Design review of the part built by this model. Coordinates are the model's own, in mm. A direction names the side the tool comes from. Coordinates: 2 decimals unless noted, no trailing zeros. Loops run counter-clockwise (first coordinate to the right, second up) from the corner with the lowest first, then second, coordinate; pieces in that order, holes last. Notation, with made-up numbers: (3, 85) -> (46, 85) arc R13 cw to (46, 100) -> close; hole circle Ø11 at (20.5, -11.75). An arc over 180 degrees is marked (long way). Answer in a Markdown table with one row per item.
```python
from build123d import *

# Parameters (mm, degrees)
BOSS_EXTRU_1_DEPTH      = 8.5
BOSS_EXTRU_1_DEPTH_BACK = 8.5
D_GAGEMENT_M41_D        = 4.8


with BuildPart() as part:
    # Esquisse1 → Boss.-Extru.1 (new, two sides: drawn at the far end of the back side and taken through both)
    with BuildSketch(Plane(origin=(0, 0, 0), x_dir=(0, 0, -1), z_dir=(1, 0, 0)).offset(-BOSS_EXTRU_1_DEPTH_BACK)):
        with BuildLine():
            Line((-3.307189139, 3.75), (-11.307189139, 3.75))
            Line((-11.307189139, 3.75), (-11.307189139, 1.75))
            Line((-11.307189139, 1.75), (-0.968245837, 1.75))
            ThreePointArc((-0.968245837, 1.75), (2, 0), (-0.968245837, -1.75))
            Line((-0.968245837, -1.75), (-11.307189139, -1.75))
            Line((-11.307189139, -1.75), (-11.307189139, -3.75))
            Line((-11.307189139, -3.75), (-3.307189139, -3.75))
            ThreePointArc((-3.307189139, -3.75), (5, 0), (-3.307189139, 3.75))
        make_face()
    extrude(amount=BOSS_EXTRU_1_DEPTH + BOSS_EXTRU_1_DEPTH_BACK)

    # Dégagement M41 (through all)
    with Locations(Plane(origin=(0, 3.75, 0), x_dir=(1, 0, 0), z_dir=(0, 1, 0))):
        with Locations((0, -7.307189139)):
            Hole(D_GAGEMENT_M41_D / 2)


solid = part.part
```
(1) Take a section at D-D on z = 0. Give the boundary of the cut face in (x, y).
Evaluation:
| item | result |
|---|---|
| outline | (-8.5, -5) -> (8.5, -5) -> (8.5, -2) -> (-8.5, -2) -> close; (-8.5, 2) -> (8.5, 2) -> (8.5, 5) -> (-8.5, 5) -> close |
(2) Take a section at B-B on z = 10.25. Give the boundary of the cut face in (x, y).
Evaluation:
| item | result |
|---|---|
| outline | (-8.5, -3.75) -> (8.5, -3.75) -> (8.5, -1.75) -> (-8.5, -1.75) -> close; (-8.5, 1.75) -> (8.5, 1.75) -> (8.5, 3.75) -> (-8.5, 3.75) -> close |
(3) Take a section at C-C on x = 4.5. Give the boundary of the cut face in (y, z), and give its area (3 significant figures).
Evaluation:
| item | result |
|---|---|
| outline | (-3.75, 3.31) arc R5 ccw (long way) to (3.75, 3.31) -> (3.75, 11.31) -> (1.75, 11.31) -> (1.75, 0.97) arc R2 cw (long way) to (-1.75, 0.97) -> (-1.75, 11.31) -> (-3.75, 11.31) -> close |
| area | 83.6 mm² |
(4) Take a section at A-A on x = 0. Give the boundary of the cut face in (y, z).
Evaluation:
| item | result |
|---|---|
| outline | (-3.75, 3.31) arc R5 ccw (long way) to (3.75, 3.31) -> (3.75, 4.91) -> (1.75, 4.91) -> (1.75, 0.97) arc R2 cw (long way) to (-1.75, 0.97) -> (-1.75, 4.91) -> (-3.75, 4.91) -> close; (-3.75, 9.71) -> (-1.75, 9.71) -> (-1.75, 11.31) -> (-3.75, 11.31) -> close; (1.75, 9.71) -> (3.75, 9.71) -> (3.75, 11.31) -> (1.75, 11.31) -> close |
(5) For pin 1 (8.5 mm diameter, centred on x = 0.5, z = 5, fed in from +Y); pin 2 (4 mm diameter, centred on x = -4, z = 9.5, fed in from -Y), all flat-tipped, find the tip position at first contact; note any pin that passes through.
Evaluation:
| item | result |
|---|---|
| pin 1 | stops at y = 4.94 |
| pin 2 | stops at y = -3.75 |
(6) To check wall thickness, follow probe 1 along Y at (x, z) = (0, 0); probe 2 along Y at (x, z) = (1.5, 4); probe 3 along X at (y, z) = (-3, 6). State the ranges of each line that lie inside material, in increasing order.
Evaluation:
| item | result |
|---|---|
| probe 1 | y = -5 to -2, 2 to 5 |
| probe 2 | y = -3.75 to -1.75, 1.75 to 3.75 |
| probe 3 | x = -8.5 to -2.01, 2.01 to 8.5 |
(7) Draft analysis for pull direction X (two halves, no side actions). For faces 1 (the cylindrical face through (0, 0, -2)), 2 (the cylindrical face through (0.52, 2.74, 9.65)), 3 (the cylindrical face through (0.52, -2.76, 9.65)), 4 (the flat face through (-8.5, -2, 3)), state which applies: pulls with the +X half, pulls with the -X half, needs draft (parallel to the pull), parting line crosses it, or undercut.
Evaluation:
| item | result |
|---|---|
| face 1 | needs draft |
| face 2 | undercut |
| face 3 | undercut |
| face 4 | pulls with the -X half |
(8) Tool access review of faces 5 (the flat face through (0, -3, 11.307)), 6 (the flat face through (-2, -3.75, 9)), 7 (the flat face through (0, -1.75, 4)), 8 (the flat face through (-2, 3.75, 5)), 9 (the cylindrical face through (0, 0, -5)): name each direction out of +Z, -Z, +X, -X, +Y, -Y from which nothing blocks a thin tool from reaching the whole face with its end or side.
Evaluation:
| item | result |
|---|---|
| face 5 | +Z, +X, -X, +Y, -Y |
| face 6 | +Z, +X, -X, -Y |
| face 7 | +Z, +X, -X |
| face 8 | +Z, +X, -X, +Y |
| face 9 | +X, -X |
